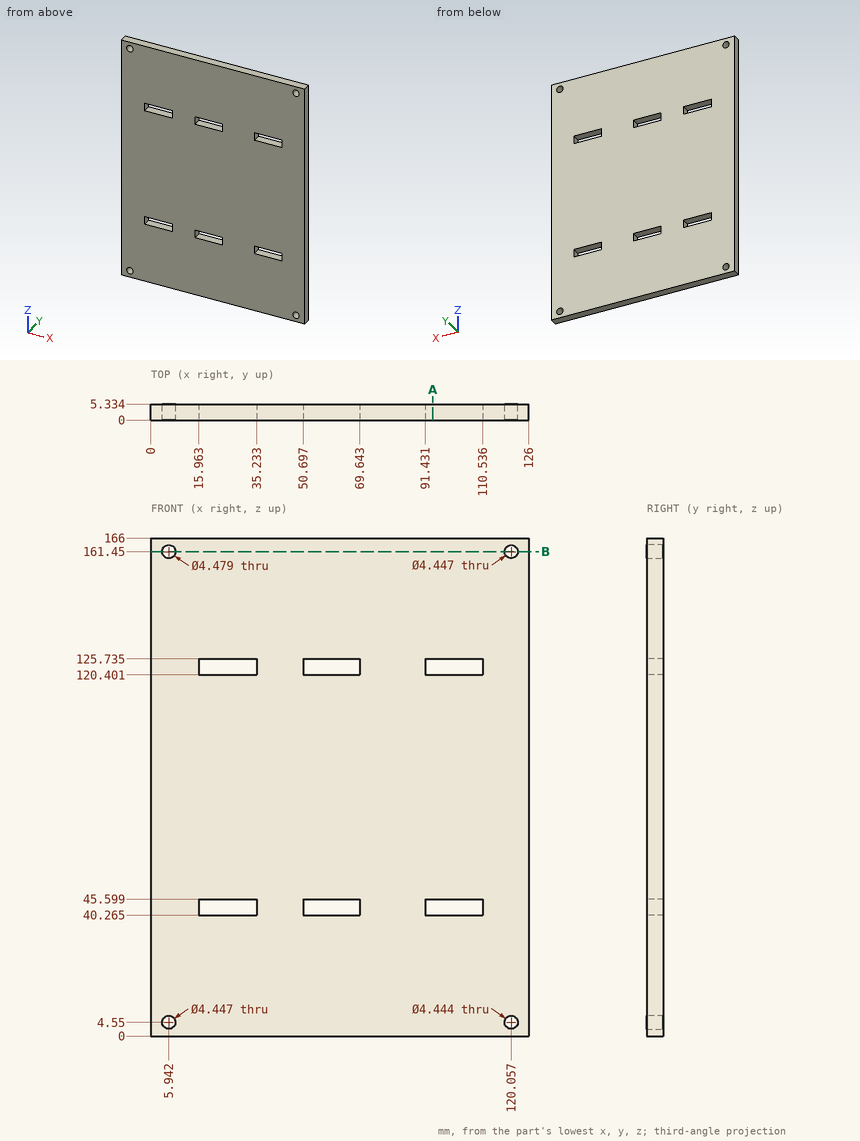
Drawing for the job (mm, zero at the part's lowest x, y, z). Round coordinates to 2 decimals unless told otherwise and drop trailing zeros. Write each loop counter-clockwise with the first axis right and the second up, starting at its lowest first coordinate (ties: lowest second). Pieces come first, ordered by that corner, then holes. Notation, with made-up numbers: M -14,14.5 L -1,14.5 A27 ccw -1,38.5 Z; hole C 65.25,78 d2. An arc over 180 degrees is marked long. Answer as a JSON object with one key per item and string values. Group by question number.
(1) Drill centre lines: L1, parallel to X at y = 3.3, z = 161.45; L2, parallel to Z at x = 30.5, y = 3.15 (1 decimal); L3, parallel to X at y = 3.45, z = 121.5 (1 decimal). Where is each one in solid material? Low to high.
(2) Cut at A-A (x = 94). Give the cut face in (y, z) (1 decimal).
(3) Cut at B-B (z = 161.45). Give the cut face in (x, y) (1 decimal).
Responses:
{
 "1": {"L1": "x = 0 to 3.7, 8.18 to 117.83, 122.28 to 126", "L2": "z = 0 to 40.3, 45.6 to 120.4, 125.7 to 166", "L3": "x = 0 to 16, 35.2 to 50.7, 69.6 to 91.4, 110.5 to 126"},
 "2": {"outline": "M 0,0 L 5.3,0 L 5.3,40.3 L 0,40.3 Z; M 0,45.6 L 5.3,45.6 L 5.3,120.4 L 0,120.4 Z; M 0,125.7 L 5.3,125.7 L 5.3,166 L 0,166 Z"},
 "3": {"outline": "M 0,0 L 3.7,0 L 3.7,5.3 L 0,5.3 Z; M 8.2,0 L 117.8,0 L 117.8,5.3 L 8.2,5.3 Z; M 122.3,0 L 126,0 L 126,5.3 L 122.3,5.3 Z"}
}
